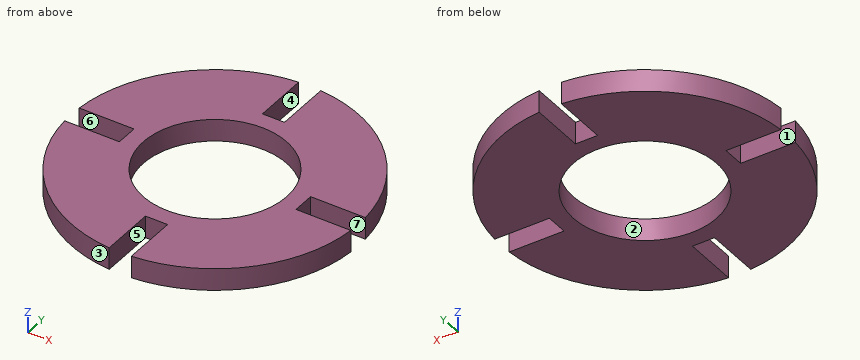
from build123d import *

# Parameters (mm, degrees)
SKETCH003_R           = 2.3
SKETCH003_W           = 2
SKETCH003_H           = 5
EXTRUDE003_DEPTH      = 5
EXTRUDE003_DEPTH_BACK = 3
ARRAY001_COUNT        = 4
SKETCH012_R           = 13
SKETCH012_R_2         = 6.5
EXTRUDE012_DEPTH      = 2


with BuildPart() as body:
    # Sketch003 → Extrude003 (new body, two sides)
    with BuildSketch(Plane.XY) as extrude003_sk:
        with Locations((0, 38.25)):
            Circle(SKETCH003_R)
        with Locations((0, 10.5)):
            Rectangle(SKETCH003_W, SKETCH003_H)
    extrude(amount=EXTRUDE003_DEPTH)
    extrude(extrude003_sk.sketch, amount=-EXTRUDE003_DEPTH_BACK)

    # Array001: Body ×4 about axis
    array001_axis = Axis((0, 0, 0), (0, 0, 1))


with BuildPart() as body_1:
    add(body.part)
    for i in range(1, ARRAY001_COUNT):
        add(body.part.rotate(array001_axis, i * 360 / ARRAY001_COUNT))


with BuildPart() as cut003:
    # Sketch012 → Extrude012 (new body)
    with BuildSketch(Plane.XY.offset(2)):
        Circle(SKETCH012_R)
        Circle(SKETCH012_R_2, mode=Mode.SUBTRACT)
    extrude(amount=-EXTRUDE012_DEPTH)

    # Cut003: cut Body
    add(body_1.part, mode=Mode.SUBTRACT)


solid = cut003.part
Part model, mm, in its own coordinate system. Face numbers are marked on the shaded views. A direction names the side the tool comes from. Give positions to 0.01 mm unless a question says otherwise; leave off trailing zeros. Loops run counter-clockwise (first coordinate to the right, second up) from the corner with the lowest first, then second, coordinate; pieces in that order, holes last. Notation, with made-up numbers: (38, -19.75) -> (59, -19.75) arc R5 cw to (59, -10.75) -> close; hole circle Ø3 at (52, 51). An arc over 180 degrees is marked (long way). Write each question's results on one line, items separated by ' | '. Start each with the question number.
Q1. Pull direction Y, two halves, no side cores. Call the marked faces 1, 2, 3 and 4: +Y half, -Y half, draft (parallel to the pull), parting line (faces both ways), or undercut.
Q2. Band-saw the part on D-D on x = 7.5. List the corners of the cut face in (y, z), plus the area to 3 significant figures.
Q3. Wall check: L1, parallel to Y at x = -0.25, z = 0.65; L2, parallel to Y at x = -10.25, z = 0.2; L3, parallel to X at y = -10, z = 0.9. Give the ranges that are in metal, low to high.
Q4. Which spindle directions (+Z, -Z, +X, -X, +Y, -Y) get a long thin tool onto all of the face, cutting with end or side? Do the marked faces 5, 6 and 7. Say none if no direction does.
Q5. Pin check, flat tips, straight feed: P1, Ø1, axis at x = 11.5, z = 1, coming from the -Y side; P2, Ø0.6, axis at y = 11, z = 0.5, coming from the +X side; P3, Ø1, axis at y = 11, z = 1, coming from the -X side. Stop position of each tip, or through.
Q6. Band-saw the part on A-A on y = 0. List the corners of the cut face in (x, z), plus the area to 3 significant figures.
Q7. Band-saw the part on C-C on z = 1. List the corners of the cut face in (x, y).
Results are:
1) face 1: undercut | face 2: undercut | face 3: -Y half | face 4: draft
2) outline: (-10.62, 0) -> (10.62, 0) -> (10.62, 2) -> (-10.62, 2) -> close | area: 42.5 mm²
3) L1: y = -8 to -6.5, 6.5 to 8 | L2: y = -8 to -1, 1 to 8 | L3: x = -8.31 to -1, 1 to 8.31
4) face 5: +Z, -Z, -Y | face 6: +Z, -Z, -X | face 7: +Z, -Z, +X
5) P1: stops at y = -6.93 | P2: stops at x = 7.38 | P3: stops at x = -7.66
6) outline: (-8, 0) -> (-6.5, 0) -> (-6.5, 2) -> (-8, 2) -> close; (6.5, 0) -> (8, 0) -> (8, 2) -> (6.5, 2) -> close | area: 6.00 mm²
7) outline: (-12.96, -1) arc R13 ccw to (-1, -12.96) -> (-1, -8) -> (1, -8) -> (1, -12.96) arc R13 ccw to (12.96, -1) -> (8, -1) -> (8, 1) -> (12.96, 1) arc R13 ccw to (1, 12.96) -> (1, 8) -> (-1, 8) -> (-1, 12.96) arc R13 ccw to (-12.96, 1) -> (-8, 1) -> (-8, -1) -> close; hole circle Ø13 at (0, 0)
